The listing builds one solid part. Answer for the finished solid, in the listing's coordinates (mm). Face numbers are marked on the shaded views. A direction names the side the tool comes from. Coordinates: 2 decimals unless noted, no trailing zeros. Return JSON: item names as keys, results as strings. Group by question number.
1. Straight lines are drawn through the part: L1, parallel to Y at x = 20.5, z = 4.5; L2, parallel to Z at x = 20.5, y = 8; L3, parallel to Z at x = 26, y = 14.25. For each, find the intervals that lie inside material, in ascending order. Write a range as from..to.
2. Which of the six approach directions +Z, -Z, +X, -X, +Y, -Y give full straight-line access (tool end or side, diameter ignored) to the marked faces 5, 6 and 7?
3. The mould has two halves that part along Y. Classify the marked faces 1, 2, 3 and 4: pulls with the +Y half, pulls with the -Y half, needs draft (parallel to the pull), parting line crosses it, or undercut.
4. Given P1, Ø6.5, axis at x = 12.5, y = 7, coming from the +Z side; P2, Ø0.5, axis at x = 19, y = 17, coming from the +Z side; P3, Ø1, axis at x = 27, z = 5, coming from the +Y side, each flat-ended and moving along its own axis, determine where each tip first touches the part or whether it passes through.
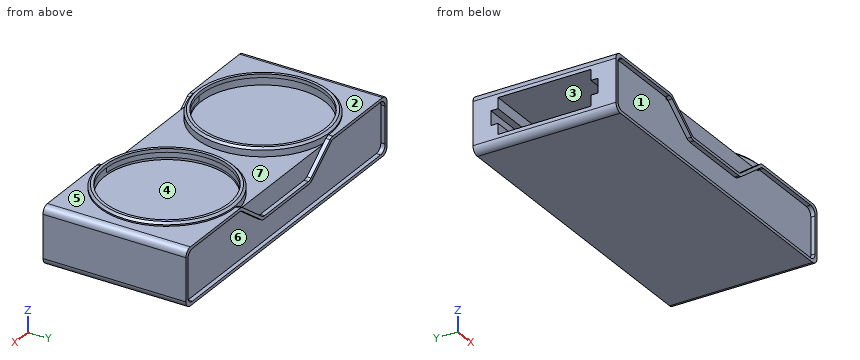
```python
from build123d import *

# Parameters (mm, degrees)
SKETCH1_W              = 45
SKETCH1_H              = 20
BOSS_EXTRUDE1_DEPTH    = 8
FILLET1_R              = 1
SKETCH3_R              = 9.4
SKETCH3_R_2            = 8.7
BOSS_EXTRUDE2_DEPTH    = 0.5
CUT_EXTRUDE1_DEPTH     = 0.6
FILLET2_R              = 1
LPATTERN3_COUNT        = 2
LPATTERN3_PITCH        = 19.4
FILLET2_OF_LPATTERN3_R = 1
SKETCH6_W              = 20.76252332
SKETCH6_H              = 18.8
CUT_EXTRUDE3_DEPTH     = 0.7
SKETCH7_R              = 9.4
SKETCH7_R_2            = 8.7
BOSS_EXTRUDE4_DEPTH    = 1.3
SKETCH8_R              = 9.4
SKETCH8_R_2            = 8.7
BOSS_EXTRUDE5_DEPTH    = 1.3
CHAMFER1_SIZE          = 0.3
SKETCH12_R             = 8.7
CUT_EXTRUDE4_DEPTH     = 1
SKETCH13_R             = 8.7
CUT_EXTRUDE5_DEPTH     = 1
SKETCH19_W             = 1.5
SKETCH19_H             = 13
SKETCH19_W_2           = 2
SKETCH19_H_2           = 1
CUT_EXTRUDE6_DEPTH     = 40


with BuildPart() as part:
    # Sketch1 → Boss-Extrude1 (new body)
    with BuildSketch(Plane.XY):
        with Locations((22.5, 10)):
            Rectangle(SKETCH1_W, SKETCH1_H)
    extrude(amount=BOSS_EXTRUDE1_DEPTH)

    # Fillet1
    fillet1_edges = [part.edges().sort_by_distance(p)[0] for p in [
        (45, 10, 8),
        (0, 10, 8),
        (45, 10, 0),
        (0, 10, 0),
    ]]
    fillet(fillet1_edges, radius=FILLET1_R)

    # Sketch3 → Boss-Extrude2 (add)
    with BuildSketch(Plane.XY.offset(8)):
        with Locations((11.75, 10)):
            Circle(SKETCH3_R)
        with Locations((11.75, 10)):
            Circle(SKETCH3_R_2, mode=Mode.SUBTRACT)
        with Locations((33.25, 10)):
            Circle(SKETCH3_R)
        with Locations((33.25, 10)):
            Circle(SKETCH3_R_2, mode=Mode.SUBTRACT)
    extrude(amount=BOSS_EXTRUDE2_DEPTH)

    # Sketch4 → Cut-Extrude1 (cut)
    with BuildSketch(Plane.XZ):
        Polygon((27.739375, 4.42), (32.55, 8), (12.45, 8), (17.260625, 4.42), align=None)
        Polygon((44.58, 7.58), (32.685625, 7.58), (27.875, 4), (27.175, 4), (17.825, 4), (17.125, 4), (12.314375, 7.58), (0.42, 7.58), (0.42, 0.42), (44.58, 0.42), align=None)
    cut_extrude1 = extrude(amount=-CUT_EXTRUDE1_DEPTH, mode=Mode.SUBTRACT)

    # Fillet2
    fillet2_edges = [part.edges().sort_by_distance(p)[0] for p in [
        (0.42, 0.3, 7.58),
        (12.314375, 0.3, 7.58),
        (17.125, 0.3, 4),
        (27.875, 0.3, 4),
        (32.685625, 0.3, 7.58),
        (44.58, 0.3, 7.58),
        (44.58, 0.3, 0.42),
        (0.42, 0.3, 0.42),
        (17.260625, 0.3, 4.42),
        (12.45, 0.3, 8),
        (32.55, 0.3, 8),
        (27.739375, 0.3, 4.42),
    ]]
    fillet(fillet2_edges, radius=FILLET2_R)

    # LPattern3: Cut-Extrude1 ×2
    with Locations(*[(0, i * LPATTERN3_PITCH, 0) for i in range(1, LPATTERN3_COUNT)]):
        add(cut_extrude1, mode=Mode.SUBTRACT)

    # Fillet2 of LPattern3
    fillet2_of_lpattern3_edges = [part.edges().sort_by_distance(p)[0] for p in [
        (0.42, 19.7, 7.58),
        (12.314375, 19.7, 7.58),
        (17.125, 19.7, 4),
        (27.875, 19.7, 4),
        (32.685625, 19.7, 7.58),
        (44.58, 19.7, 7.58),
        (44.58, 19.7, 0.42),
        (0.42, 19.7, 0.42),
        (17.260625, 19.7, 4.42),
        (12.45, 19.7, 8),
        (32.55, 19.7, 8),
        (27.739375, 19.7, 4.42),
    ]]
    fillet(fillet2_of_lpattern3_edges, radius=FILLET2_OF_LPATTERN3_R)

    # Sketch6 → Cut-Extrude3 (cut)
    with BuildSketch(Plane.XY.offset(8)):
        with Locations((22.5, 10)):
            Rectangle(SKETCH6_W, SKETCH6_H)
    extrude(amount=-CUT_EXTRUDE3_DEPTH, mode=Mode.SUBTRACT)

    # Sketch7 → Boss-Extrude4 (add)
    with BuildSketch(Plane.XY.offset(8.5)):
        with Locations((11.75, 10)):
            Circle(SKETCH7_R)
        with Locations((11.75, 10)):
            Circle(SKETCH7_R_2, mode=Mode.SUBTRACT)
    extrude(amount=-BOSS_EXTRUDE4_DEPTH)

    # Sketch8 → Boss-Extrude5 (add)
    with BuildSketch(Plane.XY.offset(8.5)):
        with Locations((33.25, 10)):
            Circle(SKETCH8_R)
        with Locations((33.25, 10)):
            Circle(SKETCH8_R_2, mode=Mode.SUBTRACT)
    extrude(amount=-BOSS_EXTRUDE5_DEPTH)

    # Chamfer1
    chamfer1_edges = [part.edges().sort_by_distance(p)[0] for p in [
        (2.35, 10, 8.5),
        (23.85, 10, 8.5),
    ]]
    chamfer(chamfer1_edges, length=CHAMFER1_SIZE)

    # Sketch12 → Cut-Extrude4 (cut)
    with BuildSketch(Plane.XY.offset(8)):
        with Locations((33.25, 10)):
            Circle(SKETCH12_R)
    extrude(amount=-CUT_EXTRUDE4_DEPTH, mode=Mode.SUBTRACT)

    # Sketch13 → Cut-Extrude5 (cut)
    with BuildSketch(Plane.XY.offset(8)):
        with Locations((11.75, 10)):
            Circle(SKETCH13_R)
    extrude(amount=-CUT_EXTRUDE5_DEPTH, mode=Mode.SUBTRACT)

    # Sketch19 → Cut-Extrude6 (cut)
    with BuildSketch(Plane.ZY):
        with Locations((5.75, 10)):
            Rectangle(SKETCH19_W, SKETCH19_H)
        with Locations((4, 10)):
            Rectangle(SKETCH19_W_2, SKETCH19_H)
        with Locations((4, 17)):
            Rectangle(SKETCH19_W_2, SKETCH19_H_2)
        with Locations((4, 3)):
            Rectangle(SKETCH19_W_2, SKETCH19_H_2)
        with Locations((2.25, 10)):
            Rectangle(SKETCH19_W, SKETCH19_H)
    extrude(amount=-CUT_EXTRUDE6_DEPTH, mode=Mode.SUBTRACT)


solid = part.part
```
Worked out:
{
 "1": {"L1": "0.6..2.5, 17.5..19.4", "L2": "0..1.5, 6.5..8.5", "L3": "0..1.5, 6.5..7"},
 "2": {"face 5": "+Z, +X", "face 6": "+Y", "face 7": "+Z"},
 "3": {"face 1": "pulls with the -Y half", "face 2": "needs draft", "face 3": "undercut", "face 4": "undercut"},
 "4": {"P1": "z = 7", "P2": "z = 7.3", "P3": "y = 19.4"}
}
